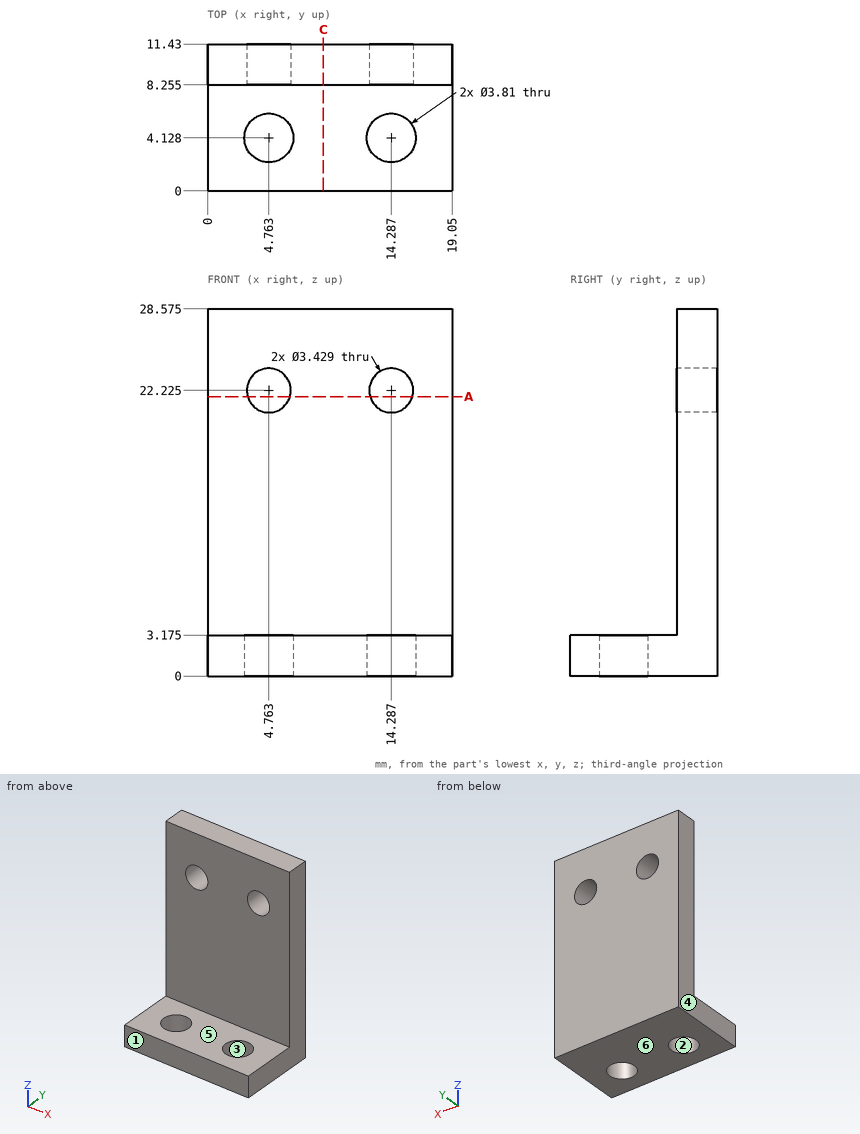
Job drawing, mm, ordinate dimensions from the low corner. One solid piece. A direction names the side the tool comes from. Round coordinates to 2 decimals unless told otherwise and drop trailing zeros. Write each loop counter-clockwise with the first axis right and the second up, starting at its lowest first coordinate (ties: lowest second). Pieces come first, ordered by that corner, then holes. Notation, with made-up numbers: (76.5, 20) -> (106.5, 20) arc R16 cw to (106.5, 31) -> close; hole circle Ø8 at (3.5, 72.25). An arc over 180 degrees is marked (long way). Answer as CSV lines item,"result".
1. Mould opens along Y. For the marked faces 1, 2, 3 and 4 say: +Y half, -Y half, draft (parallel to the pull), parting line (faces both ways), or undercut.
Resolved:
face 1,"-Y half"
face 2,"undercut"
face 3,"undercut"
face 4,"draft"
2. Tool access for the marked faces 5 and 6: list every direction of +Z, -Z, +X, -X, +Y, -Y with a clear straight run to the whole face (end or side of a thin tool).
Resolved:
face 5,"+Z, +X, -X, -Y"
face 6,"-Z, +X, -X, +Y, -Y"
3. Pin check, flat tips, straight feed: pin 1 Ø4.5 at (x, z) = (14.29, 22.22) entering from +Y; pin 2 Ø1 at (y, z) = (7.5, 14.5) entering from +X; pin 3 Ø9.5 at (x, z) = (10, 12) entering from -Y (1 decimal); pin 4 Ø1.5 at (x, y) = (2, 6.5) entering from +Z (1 decimal). Stop position of each tip, or through.
Resolved:
pin 1,"y = 11.43"
pin 2,"through"
pin 3,"y = 8.3"
pin 4,"z = 3.2"
4. Slice it at A-A, the plane z = 21.75. State how many separate pieces and enclosed holes the cut face has.
Resolved:
separate pieces,"3"
enclosed holes,"0"
5. Slice it at C-C, the plane x = 9. List the corners of the cut face in (y, z) (1 decimal), plus the area to 3 significant figures.
Resolved:
outline,"(0, 0) -> (11.4, 0) -> (11.4, 28.6) -> (8.3, 28.6) -> (8.3, 3.2) -> (0, 3.2) -> close"
area,"117 mm²"
6. Drill centre lines: line 1 (X direction, y = 10.75, z = 22.25); line 2 (Y direction, x = 15.25, z = 10.5) (1 decimal); line 3 (Z direction, x = 15, y = 7.5) (1 decimal). Where is each one in solid material? Low to high.
Resolved:
line 1,"0 to 3.05, 6.48 to 12.57, 16 to 19.05"
line 2,"8.3 to 11.4"
line 3,"0 to 3.2"
